from build123d import *

# Parameters (mm, degrees)
F2_DEPTH = 8.4
F4_R     = 0.2


with BuildPart() as f2:
    # F1 (on Top) → F2 (new body)
    with BuildSketch(Plane.XY):
        Polygon((-31.005243456, 25.9445533505), (-32.9355241115, 25.4210874101), (-31.6268592603, 20.5953857712), (-29.6965786048, 21.1188517117), align=None)
    extrude(amount=F2_DEPTH)

    # F3: F2 across plane


with BuildPart() as f2_1:
    add(f2.part)
    add(f2.part.mirror(Plane.XY))

    # F4
    f4_edges = [f2_1.edges().sort_by_distance(p)[0] for p in [
        (-30.661719, 20.857119, 8.4),
        (-30.350911, 23.531703, 8.4),
        (-31.970384, 25.68282, 8.4),
        (-32.281192, 23.008237, 8.4),
        (-31.626859, 20.595386, 0),
        (-29.696579, 21.118852, 0),
        (-30.661719, 20.857119, -8.4),
        (-32.935524, 25.421087, 0),
        (-31.970384, 25.68282, -8.4),
        (-31.005243, 25.944553, 0),
        (-30.350911, 23.531703, -8.4),
        (-32.281192, 23.008237, -8.4),
    ]]
    fillet(f4_edges, radius=F4_R)


solid = f2_1.part
Read the model definition and answer for the solid it produces. Units are mm, in the model's axes. Give positions to 0.01 mm unless a question says otherwise; leave off trailing zeros. Write each loop counter-clockwise with the first axis right and the second up, starting at its lowest first coordinate (ties: lowest second). Pieces come first, ordered by that corner, then holes. Notation, with made-up numbers: (-37.5, -38) - (-18.5, -38) arc R13 ccw to (-18.5, -21) - close; hole circle Ø2 at (-10, 53). An arc over 180 degrees is marked (long way). Return JSON: item names as keys, results as strings.
Q1. A cutting plane is placed at A-A, the plane z = -1. Determine the outline of the cut face in (x, y).
Reply:
{"outline": "(-32.88, 25.23) - (-31.68, 20.79) arc R0.2 ccw to (-31.43, 20.65) - (-29.89, 21.07) arc R0.2 ccw to (-29.75, 21.31) - (-30.95, 25.75) arc R0.2 ccw to (-31.2, 25.89) - (-32.74, 25.47) arc R0.2 ccw to start"}
Q2. Given P1, Ø1, axis at y = 21.5, z = 1.5, coming from the -X side, flat-ended and moving along its own axis, determine where the tip first touches the part or whether it passes through.
Reply:
{"P1": "x = -32.01"}
Q3. Consider line 1 along Y through (x, z) = (-31.2, 1.25); line 2 along X through (y, z) = (23.4, -7.25); line 3 along X through (y, z) = (22.65, -6). Determine where each line is inside the solid, lowest interval first. Write a range as [from, to].
Reply:
{"line 1": "[20.71, 25.89]", "line 2": "[-32.39, -30.32]", "line 3": "[-32.18, -30.11]"}
